from build123d import *

# Parameters (mm, degrees)
SKETCH1_W           = 70
SKETCH1_H           = 60
BOSS_EXTRUDE1_DEPTH = 45
SKETCH2_W           = 42
SKETCH2_H           = 27
CUT_EXTRUDE1_DEPTH  = 103.591422643
SKETCH3_R           = 16
CUT_EXTRUDE2_DEPTH  = 45
SKETCH4_W           = 25
SKETCH4_H           = 25
CUT_EXTRUDE3_DEPTH  = 25
FILLET1_R           = 10
FILLET2_R           = 5
SKETCH9_R           = 5
CUT_EXTRUDE4_DEPTH  = 103.591422643


with BuildPart() as part:
    # Sketch1 → Boss-Extrude1 (new body)
    with BuildSketch(Plane(origin=(0, 0, 0), x_dir=(1, 0, 0), z_dir=(0, 1, 0))):
        with Locations((35, 30)):
            Rectangle(SKETCH1_W, SKETCH1_H)
    extrude(amount=BOSS_EXTRUDE1_DEPTH)

    # Sketch2 → Cut-Extrude1 (cut, through all)
    with BuildSketch(Plane(origin=(70, 0, 0), x_dir=(0, 0, -1), z_dir=(1, 0, 0))):
        with Locations((39, 13.5)):
            Rectangle(SKETCH2_W, SKETCH2_H)
    extrude(amount=-CUT_EXTRUDE1_DEPTH, mode=Mode.SUBTRACT)

    # Sketch3 → Cut-Extrude2 (cut)
    with BuildSketch(Plane(origin=(0, 45, 0), x_dir=(1, 0, 0), z_dir=(0, 1, 0))):
        with Locations((35, 55)):
            Circle(SKETCH3_R)
    extrude(amount=-CUT_EXTRUDE2_DEPTH, mode=Mode.SUBTRACT)

    # Sketch4 → Cut-Extrude3 (cut)
    with BuildSketch(Plane.XY):
        with Locations((35, 32.5)):
            Rectangle(SKETCH4_W, SKETCH4_H)
    extrude(amount=-CUT_EXTRUDE3_DEPTH, mode=Mode.SUBTRACT)

    # Fillet1
    fillet1_edges = [part.edges().sort_by_distance(p)[0] for p in [
        (58.75, 45, 0),
        (11.25, 45, 0),
    ]]
    fillet(fillet1_edges, radius=FILLET1_R)

    # Fillet2
    fillet2_edges = [part.edges().sort_by_distance(p)[0] for p in [
        (11.25, 27, -18),
        (58.75, 27, -18),
    ]]
    fillet(fillet2_edges, radius=FILLET2_R)

    # Sketch9 → Cut-Extrude4 (cut, through all)
    with BuildSketch(Plane(origin=(70, 0, 0), x_dir=(0, 0, -1), z_dir=(1, 0, 0))):
        with Locations((10, 35)):
            Circle(SKETCH9_R)
    extrude(amount=-CUT_EXTRUDE4_DEPTH, mode=Mode.SUBTRACT)


solid = part.part
Check sheet for the modelled part. Datum: model origin and axes. Units: mm. A direction names the side the tool comes from. Give positions to 0.01 mm unless a question says otherwise; leave off trailing zeros. Order: outer loops, then holes, each group sorted by start corner. A loop starts at its lowest first (then second) coordinate and runs counter-clockwise, first axis right, second up. Notation, with made-up numbers: M 52,-6.75 L 91,-6.75 A15 cw 91,17.25 Z; hole C 19,53.25 d9. An arc over 180 degrees is marked long. Answer as CSV lines item,"result". Start each with the question number.
Item 1: Cross-section at A-A on z = -24. Enter the section's corners in (x, y), plus the area to 3 significant figures.
Item 2: Thickness scan on line 1 (X direction, y = 39, z = -55); line 2 (X direction, y = 34.5, z = -16); line 3 (Z direction, x = 35, y = 33). Record the ranges inside material, lowest first. Write a range as [from, to].
Item 3: Tool access check on faces 4 (the face through (35, 20, -9)), 5 (the face through (35, 11, -18)), 6 (the face through (35, 36, -25)), 7 (the face through (22.5, 30, -12)). Record the directions out of +Z, -Z, +X, -X, +Y, -Y that give a thin tool (end or side, any length) a straight path to the whole face; none if there is none.
Item 4: Cross-section at B-B on x = 35. Enter the section's corners in (y, z), plus the area to 3 significant figures.
Item 5: Cross-section at C-C on y = 41. Enter the section's corners in (x, z).
Item 6: Mould release check, pull along X, two halves, no side actions. Record for faces 1 (the face through (10, 36, -60)), 2 (the face through (70, 27.2, -22.9)), 3 (the face through (35, 36, -39)): +X half, -X half, draft (parallel to the pull), parting line (faces both ways), or undercut.
Item 7: Cross-section at D-D on z = -9. Enter the section's corners in (x, y), plus the area to 3 significant figures.
Item 8: Gauge pin test, flat ends, axial feed: P1, Ø20, axis at x = 35.5, y = 34.5, coming from the +Z side; P2, Ø9, axis at x = 31, z = -7.5, coming from the +Y side; P3, Ø8, axis at x = 52.5, z = -29, coming from the -Y side; P4, Ø9, axis at y = 35, z = -10, coming from the -X side. Record the tip position at first contact, or that the pin passes through.
Established:
1,outline,"M 0,27 L 22.5,27 L 22.5,45 L 0,45 Z; M 47.5,27 L 70,27 L 70,45 L 47.5,45 Z"
1,area,"810 mm^2"
2,line 1,"x = [0, 19], [51, 70]"
2,line 2,"x = [0, 22.5], [47.5, 70]"
2,line 3,"z = [-39, -25]"
3,face 4,"+Z, -Z, +Y"
3,face 5,"-Z, +X, -X, -Y"
3,face 6,"+Z, +Y, -Y"
3,face 7,"+Z, +Y"
4,outline,"M 0,-18 L 20,-18 L 20,0 L 0,0 Z; M 27,-39 L 45,-39 L 45,-25 L 27,-25 Z"
4,area,"612 mm^2"
5,outline,"M 0,-60 L 19.8,-60 A16 cw long 50.2,-60 L 70,-60 L 70,-2 L 47.5,-2 L 47.5,-25 L 22.5,-25 L 22.5,-2 L 0,-2 Z"
6,face 1,"draft"
6,face 2,"+X half"
6,face 3,"undercut"
7,outline,"M 0,0 L 70,0 L 70,30.1 L 47.5,30.1 L 47.5,20 L 22.5,20 L 22.5,30.1 L 0,30.1 Z; M 0,39.9 L 22.5,39.9 L 22.5,44.95 L 0,44.95 Z; M 47.5,39.9 L 70,39.9 L 70,44.95 L 47.5,44.95 Z"
7,area,"2,080 mm^2"
8,P1,"stops at z = -25"
8,P2,"stops at y = 20"
8,P3,"stops at y = 27"
8,P4,"passes through"
